Could you check a few things on this model? Use its own coordinates, in mm. A direction names the side the tool comes from. Round coordinates to 2 decimals unless told otherwise and drop trailing zeros.
from build123d import *

# Parameters (mm, degrees)
MAINBASESKETCH_W                 = 23.8
MAINBASESKETCH_H                 = 3.2
MAINBASEEXTRUDE_DEPTH            = 11.9
STUDSSKETCH_R                    = 2.31
STUDSEXTRUDE_DEPTH               = 1.6
STUDSPATTERN_COUNT               = 3
STUDSPATTERN_PITCH               = 8
STUDSPATTERN_COUNT_DIR2          = 3
STUDSPATTERN_PITCH_DIR2          = 8
MAINBASESHELL_T                  = -1.2
TABLEBASEUNDERCIRCLES_START      = -0.2
TABLEBASEUNDERCIRCLESKETCHES_R   = 3.1
TABLEBASEUNDERCIRCLESKETCHES_R_2 = 2.4
TABLEBASEUNDERCIRCLES_DEPTH      = 2.4


with BuildPart() as part:
    # MainBaseSketch → MainBaseExtrude (new, symmetric)
    with BuildSketch(Plane.XY):
        with Locations((12.581967213, 1.6)):
            Rectangle(MAINBASESKETCH_W, MAINBASESKETCH_H)
    extrude(amount=MAINBASEEXTRUDE_DEPTH, both=True)

    # StudsSketch → StudsExtrude (add)
    with BuildSketch(Plane(origin=(0, 3.2, 0), x_dir=(1, 0, 0), z_dir=(0, 1, 0))):
        with Locations((4.581967213, 8)):
            Circle(STUDSSKETCH_R)
    studsextrude = extrude(amount=STUDSEXTRUDE_DEPTH)

    # StudsPattern: StudsExtrude 3 × 3
    with Locations(*[(j * STUDSPATTERN_PITCH_DIR2, 0, i * STUDSPATTERN_PITCH) for i in range(STUDSPATTERN_COUNT) for j in range(STUDSPATTERN_COUNT_DIR2) if (i, j) != (0, 0)]):
        add(studsextrude)

    # MainBaseShell
    mainbaseshell_openings = [part.faces().sort_by_distance(p)[0] for p in [
        (12.581967213, 0, 0),
    ]]
    offset(amount=MAINBASESHELL_T, openings=mainbaseshell_openings, kind=Kind.INTERSECTION)

    # TableBaseUnderCircleSketches → TableBaseUnderCircles (add)
    # profile 1 of 4: a face of its own
    with BuildSketch(Plane.XZ.offset(-2).offset(TABLEBASEUNDERCIRCLES_START)):
        with Locations((8.581967213, 4)):
            Circle(TABLEBASEUNDERCIRCLESKETCHES_R)
        with Locations((8.581967213, 4)):
            Circle(TABLEBASEUNDERCIRCLESKETCHES_R_2, mode=Mode.SUBTRACT)
    # profile 2 of 4: a face of its own
    with BuildSketch(Plane.XZ.offset(-2).offset(TABLEBASEUNDERCIRCLES_START)):
        with Locations(Location((16.581967213, 4, 0), (0, 0, 90))):
            Circle(TABLEBASEUNDERCIRCLESKETCHES_R)
        with Locations(Location((16.581967213, 4, 0), (0, 0, 90))):
            Circle(TABLEBASEUNDERCIRCLESKETCHES_R_2, mode=Mode.SUBTRACT)
    # profile 3 of 4: a face of its own
    with BuildSketch(Plane.XZ.offset(-2).offset(TABLEBASEUNDERCIRCLES_START)):
        with Locations(Location((8.581967213, -4, 0), (0, 0, 90))):
            Circle(TABLEBASEUNDERCIRCLESKETCHES_R)
        with Locations(Location((8.581967213, -4, 0), (0, 0, 90))):
            Circle(TABLEBASEUNDERCIRCLESKETCHES_R_2, mode=Mode.SUBTRACT)
    # profile 4 of 4: a face of its own
    with BuildSketch(Plane.XZ.offset(-2).offset(TABLEBASEUNDERCIRCLES_START)):
        with Locations(Location((16.581967213, -4, 0), (0, 0, 90))):
            Circle(TABLEBASEUNDERCIRCLESKETCHES_R)
        with Locations(Location((16.581967213, -4, 0), (0, 0, 90))):
            Circle(TABLEBASEUNDERCIRCLESKETCHES_R_2, mode=Mode.SUBTRACT)
    extrude(amount=TABLEBASEUNDERCIRCLES_DEPTH)


solid = part.part
Item 1: If we section it at A-A, the plane y = 4.25: Count the separate pieces of the cut face and the enclosed holes in it, then the cut area to 3 significant figures.
Results list:
separate pieces: 9
enclosed holes: 0
area: 151 mm2
Item 2: For faces 1 (the flat face through (13, 4.8, 0)), 2 (the cylindrical face through (19.473, 2.789, -0.049)), 3 (the cylindrical face through (18.75, 3.99, -6.59)), which set-ups out of +Z, -Z, +X, -X, +Y, -Y let a thin tool reach every point of the face, with its end or its side?
Results list:
face 1: +Z, -Z, +X, -X, +Y
face 2: -Y
face 3: +Y
Item 3: Will these pins go through, and if not, where does the flat tip stop? pin 1 (1.3 mm diameter, centred on x = 12.58, z = -8, fed in from -Y); pin 2 (1.8 mm diameter, centred on x = 13, z = 0, fed in from -Y).
Results list:
pin 1: stops at y = 3.6
pin 2: stops at y = 2
Item 4: If I drill on line 1 along X through (y, z) = (1.3, -4); line 2 along Z through (x, y) = (20.5, 2.8); line 3 along Z through (x, y) = (21.75, 1.1), over which ranges is the centre line in solid material (lowest first)?
Results list:
line 1: x = 0.68 to 1.88, 5.48 to 6.18, 10.98 to 11.68, 13.48 to 14.18, 18.98 to 19.68, 23.28 to 24.48
line 2: z = -11.9 to -9.11, -6.89 to -1.11, 1.11 to 6.89, 9.11 to 11.9
line 3: z = -11.9 to -10.7, 10.7 to 11.9
Item 5: We'd pull the mould along X, two halves only. Please class faces 4 (the flat face through (12, 2, 3)), 5 (the flat face through (21, 4.8, -8)): released by +X, released by -X, zero draft, split by the parting line, or undercut.
Results list:
face 4: undercut
face 5: zero draft
